from build123d import *

# Parameters (mm, degrees)
F0_W      = 80
F0_H      = 80
F1_DEPTH  = 5
F2_W      = 15
F2_H      = 15
F3_DEPTH  = 20
F6_D      = 7.5
F9_D      = 7.5
F10_R     = 2.75
F11_DEPTH = 15


with BuildPart() as f1:
    # F0 (on Top) → F1 (new body)
    with BuildSketch(Plane.XY):
        Rectangle(F0_W, F0_H)
    extrude(amount=F1_DEPTH)

    # F2 (on Top) → F3 (join)
    with BuildSketch(Plane.XY):
        with Locations((-32.3208275437, 0.3642106242)):
            Rectangle(F2_W, F2_H)
        with Locations((32.3208275437, 0.3642106242)):
            Rectangle(F2_W, F2_H)
        with Locations((0.3983431309, -32.6577353477)):
            Rectangle(F2_W, F2_H)
        with Locations((0.3983431309, 32.6577353477)):
            Rectangle(F2_W, F2_H)
    extrude(amount=-F3_DEPTH)

    # F6 (through all)
    with Locations(Plane.XZ.offset(41.1)):
        with Locations((0, -10.4419896379)):
            Hole(F6_D / 2)

    # F9 (through all)
    with Locations(Plane.YZ.offset(59.3)):
        with Locations((0, -10.4419896379)):
            Hole(F9_D / 2)

    # F10 (on Top) → F11 (join)
    with BuildSketch(Plane.XY):
        with Locations((-32.6312184334, 29.5856371522)):
            Circle(F10_R)
        with Locations((32.6312184334, 29.5856371522)):
            Circle(F10_R)
        with Locations((32.6312184334, -29.5856371522)):
            Circle(F10_R)
        with Locations((-32.6312184334, -29.5856371522)):
            Circle(F10_R)
    extrude(amount=-F11_DEPTH)


solid = f1.part
Work out the finished part from the listing and answer in its coordinate system (mm). A direction names the side the tool comes from. Give positions to 0.01 mm unless a question says otherwise; leave off trailing zeros. Loops run counter-clockwise (first coordinate to the right, second up) from the corner with the lowest first, then second, coordinate; pieces in that order, holes last. Notation, with made-up numbers: (63.5, 28.25) -> (105.5, 28.25) arc R7 cw to (105.5, 32.25) -> close; hole circle Ø4 at (-31, 30). An arc over 180 degrees is marked (long way). Use a Markdown table: item, result. Add a question column.
1. Flat-ended cylindrical pins translate along their axes: pin 1 Ø4.5 at (y, z) = (1, -6.5) entering from -X; pin 2 Ø12 at (y, z) = (32.5, -7.5) entering from +X; pin 3 Ø6 at (x, y) = (33, -29.5) entering from -Z. Find the tip coordinate at first contact, or state that the pin passes through.
2. Determine the mould class of faces 1 (the flat face through (-39.821, 4, -8)), 2 (the flat face through (33, 30, -15)), 3 (the cylindrical face through (34.11, -27.267, -7.395)) for opening direction X: released by +X, released by -X, zero draft, split by the parting line, or undercut.
3. Find the intervals of material crossed by probe 1 along Y at (x, z) = (-2, -16.25); probe 2 along X at (y, z) = (5.5, -5); probe 3 along Z at (x, y) = (0, -35.5), in increasing order.
4. Section B-B on y = 0 is taken. Determine the outline of the cut face in (x, z).
5. Section A-A on x = 0 is taken. Determine the outline of the cut face in (y, z).
6. For faces 4 (the flat face through (-32, -7.136, -10)), 5 (the flat face through (-24.821, 4, -8)), 6 (the cylindrical face through (-35.38, 29.71, -7.4)), determine the directions among +Z, -Z, +X, -X, +Y, -Y from which every point of the face is accessible in a straight line to the end or side of a thin tool.
7. Section D-D on x = -15 is taken. Determine the outline of the cut face in (y, z).
8. Section C-C on y = 34 is taken. Determine the outline of the cut face in (x, z), and give its area (3 significant figures).
Results below:
| question | item | result |
|---|---|---|
| 1 | pin 1 | stops at x = -39.82 |
| 1 | pin 2 | stops at x = 35.38 |
| 1 | pin 3 | stops at z = -15 |
| 2 | face 1 | released by -X |
| 2 | face 2 | zero draft |
| 2 | face 3 | undercut |
| 3 | probe 1 | y = -40.16 to -25.16, 25.16 to 40.16 |
| 3 | probe 2 | x = -39.82 to -24.82, 24.82 to 39.82 |
| 3 | probe 3 | z = -20 to -14.19, -6.69 to 5 |
| 4 | outline | (-40, 0) -> (-39.82, 0) -> (-39.82, -6.69) -> (-24.82, -6.69) -> (-24.82, 0) -> (24.82, 0) -> (24.82, -6.69) -> (39.82, -6.69) -> (39.82, 0) -> (40, 0) -> (40, 5) -> (-40, 5) -> close; (-39.82, -20) -> (-24.82, -20) -> (-24.82, -14.19) -> (-39.82, -14.19) -> close; (24.82, -20) -> (39.82, -20) -> (39.82, -14.19) -> (24.82, -14.19) -> close |
| 5 | outline | (-40.16, -20) -> (-25.16, -20) -> (-25.16, -14.19) -> (-40.16, -14.19) -> close; (-40.16, -6.69) -> (-25.16, -6.69) -> (-25.16, 0) -> (25.16, 0) -> (25.16, -6.69) -> (40.16, -6.69) -> (40.16, 0) -> (40, 0) -> (40, 5) -> (-40, 5) -> (-40, 0) -> (-40.16, 0) -> close; (25.16, -20) -> (40.16, -20) -> (40.16, -14.19) -> (25.16, -14.19) -> close |
| 6 | face 4 | -Z, +X, -X |
| 6 | face 5 | -Z, +Y, -Y |
| 6 | face 6 | -Z |
| 7 | outline | (-40, 0) -> (40, 0) -> (40, 5) -> (-40, 5) -> close |
| 8 | outline | (-40, 0) -> (-7.1, 0) -> (-7.1, -20) -> (7.9, -20) -> (7.9, 0) -> (40, 0) -> (40, 5) -> (-40, 5) -> close; hole circle Ø7.5 at (0, -10.44) |
| 8 | area | 656 mm^2 |
